Check sheet for the modelled part. Datum: model origin and axes. Units: mm. Face numbers are marked on the shaded views. A direction names the side the tool comes from. Give positions to 0.01 mm unless a question says otherwise; leave off trailing zeros. Order: outer loops, then holes, each group sorted by start corner. A loop starts at its lowest first (then second) coordinate and runs counter-clockwise, first axis right, second up.
Autodesk Inventor part; units mm, degrees
ref_plane "YZ Plane" through (0, 0, 0) normal (1, 0, 0) x (0, 1, 0)
ref_plane "XZ Plane" through (0, 0, 0) normal (0, 1, 0) x (-1, 0, 0)
ref_plane "XY Plane" through (0, 0, 0) normal (0, 0, 1) x (1, 0, 0)
sketch "Sketch1" plane through (0, 0, 0) normal (0, 1, 0) x (-1, 0, 0)
  line L0 (-40, -47.5) -> (40, -47.5)
  line L1 (40, -47.5) -> (40, 47.5)
  line L2 (40, 47.5) -> (-40, 47.5)
  line L3 (-40, 47.5) -> (-40, -47.5)
  line L4 (-40, -47.5) -> (40, 47.5) construction
  line L5 (40, -47.5) -> (-40, 47.5) construction
  line L6 (25.5, 17) -> (28.5, 17)
  line L7 (0, 17.5) -> (0, 19)
  line L8 (0, 0) -> (2.25, 0)
  line L9 (0, 0) -> (0, 17.5)
  line L10 (-27.5, -36.75) -> (-27.5, 38.25)
  line L11 (-27.5, 38.25) -> (28.5, -36.75) construction
  line L12 (28.5, 38.25) -> (-27.5, -36.75) construction
  line L13 (28.5, 38.25) -> (28.5, -36.75)
  line L14 (28.5, 17) -> (28.5, -36.75)
  line L15 (28.5, -36.75) -> (-27.5, -36.75)
  line L16 (0, -31.5) -> (8.5, -31.5)
  line L17 (0, 0) -> (0, -31.5)
  line L18 (0, -31.5) -> (-19.5, -31.5)
  line L19 (-19.5, -31.5) -> (-19.5, -36.75)
  line L20 (-27.5, 38.25) -> (28.5, 38.25)
  line L21 (0, 19) -> (24, 19)
  line L22 (0, 0) -> (0, 31.5)
  line L23 (28.5, -17) -> (28.5, 36.75)
  line L24 (28.5, -38.25) -> (28.5, 36.75)
  line L25 (28.5, -38.25) -> (-27.5, 36.75) construction
  line L26 (-27.5, 36.75) -> (-27.5, -38.25)
  line L27 (-27.5, -38.25) -> (28.5, 36.75) construction
  line L28 (0, 31.5) -> (8.5, 31.5)
  circle A0 centre (8.5, 31.5) radius 2.5
  line L29 (0, 31.5) -> (-19.5, 31.5)
  circle A1 centre (-19.5, 31.5) radius 2.5
  circle A2 centre (-19.5, 31.5) radius 2.5
  line L30 (-19.5, 31.5) -> (-19.5, 36.75)
  line L31 (28.5, 36.75) -> (-27.5, 36.75)
  line L32 (0, 0) -> (0, -17.5)
  line L33 (0, -17.5) -> (0, -19)
  line L34 (25.5, -17) -> (28.5, -17)
  line L35 (0, -19) -> (24, -19)
  line L36 (-27.5, -38.25) -> (28.5, -38.25)
  circle A3 centre (24, -19) radius 2.5
  point P0 (0.5, 0.75)
  point P1 (0.5, -0.75)
  dimension "d0" = 80
  dimension "d1" = 95
  dimension "d5" = 17.5
  dimension "d6" = 8.5
  dimension "d7" = 19.5
  dimension "d8" = 31.5
  dimension "d9" = 24
  dimension "d11" = 2.25
  dimension "d12" = 56
  dimension "d13" = 75
  dimension "d14" = 5.25
  dimension "d15" = 3
ref_plane "Work Plane3" through (0, 10, 0) normal (0, 1, 0) x (1, 0, 0)
sketch "Sketch2" plane through (0, 10, 0) normal (0, 1, 0) x (1, 0, 0)
  line L0 (35.5, -47.5) -> (40, -39.7058)
  line L1 (35.5, -47.5) -> (44.5, -47.5) construction
  line L2 (40, -39.7058) -> (35.5, -39.7058)
  line L3 (35.5, -39.7058) -> (35.5, -47.5)
  line L4 (-40, -47.5) -> (40, -47.5)
  line L5 (40, -47.5) -> (40, 47.5)
  line L6 (40, -37.7058) -> (33.5, -37.7058)
  line L7 (33.5, -37.7058) -> (33.5, -47.5)
  line L8 (33.5, -47.5) -> (35.5, -47.5)
  line L9 (40, -39.7058) -> (40, -37.7058)
  line L10 (0, -47.5) -> (0, 47.5)
  line L11 (-35.5, -47.5) -> (-40, -39.7058)
  line L12 (-35.5, -47.5) -> (-44.5, -47.5) construction
  line L13 (-40, -39.7058) -> (-35.5, -39.7058)
  line L14 (-35.5, -39.7058) -> (-35.5, -47.5)
  line L15 (-40, -37.7058) -> (-33.5, -37.7058)
  line L16 (-33.5, -37.7058) -> (-33.5, -47.5)
  line L17 (-33.5, -47.5) -> (-35.5, -47.5)
  line L18 (-40, -39.7058) -> (-40, -37.7058)
  line L19 (40, 47.5) -> (-40, 47.5)
  line L20 (-40, 47.5) -> (-33.5, 47.5)
  line L21 (-33.5, 47.5) -> (-33.5, 37.5)
  line L22 (-33.5, 37.5) -> (-40, 37.5)
  line L23 (-40, 37.5) -> (-40, 47.5)
  line L24 (40, 47.5) -> (33.5, 47.5)
  line L25 (33.5, 47.5) -> (33.5, 37.5)
  line L26 (33.5, 37.5) -> (40, 37.5)
  line L27 (40, 37.5) -> (40, 47.5)
  point P0 (0, 0)
  dimension "d18" = 9
  dimension "d19" = 60
  dimension "d20" = 2
  dimension "d21" = 9.7942
  dimension "d22" = 6.5
  dimension "d23" = 6.5
  dimension "d24" = 10
  dimension "d25" = 6.5
  dimension "d26" = 10
extrude "Extrusion2" add sketch "Sketch2" along normal blind 100 contours L3 L2 L0 | L4 L7 L6 L5 L2 L3 | L26 L25 L19 L5 | L14 L13 L18 L15 L16 L4 | L11 L13 L14 | L21 L22 L23 L19
ref_plane "Work Plane2" through (0, 10, 0) normal (0, 1, 0) x (1, 0, 0)
sketch "Sketch3" plane through (0, 10, 0) normal (0, 1, 0) x (1, 0, 0)
  line L0 (-40, 37.5) -> (-40, -37.7058)
  line L1 (-33.5, 37.5) -> (-40, 37.5)
  line L2 (-40, -37.7058) -> (-36.75, -37.7058)
  line L3 (-36.75, -37.7058) -> (-36.75, 37.5)
  line L4 (-36.75, 37.5) -> (-40, 37.5)
  line L5 (-40, 37.5) -> (-40, -37.7058)
  line L6 (33.5, 37.5) -> (40, 37.5)
  line L7 (40, -37.7058) -> (33.5, -37.7058)
  line L8 (40, 37.5) -> (36.75, 37.5)
  line L9 (36.75, 37.5) -> (36.75, -37.7058)
  line L10 (36.75, -37.7058) -> (40, -37.7058)
  line L11 (40, -37.7058) -> (40, 37.5)
  point P0 (0, 0)
extrude "Extrusion3" add sketch "Sketch3" along normal blind 5
ref_plane "Work Plane4" through (0, 110, 0) normal (0, 1, 0) x (1, 0, 0)
sketch "Sketch4" plane through (0, 110, 0) normal (0, 1, 0) x (1, 0, 0)
  line L0 (-33.5, 47.5) -> (-40, 47.5)
  line L1 (-40, -47.5) -> (40, -47.5)
  line L2 (-40, 47.5) -> (-33.5, 47.5)
  line L3 (-33.5, 47.5) -> (-33.5, -47.5)
  line L4 (-33.5, -47.5) -> (-40, -47.5)
  line L5 (-40, -47.5) -> (-40, 47.5)
  line L6 (40, 37.5) -> (40, 47.5)
  line L7 (40, 47.5) -> (33.5, 47.5)
  line L8 (33.5, 47.5) -> (33.5, -47.5)
  line L9 (33.5, -47.5) -> (40, -47.5)
  line L10 (40, -47.5) -> (40, 47.5)
  line L11 (40, -37.7058) -> (33.5, -37.7058)
  line L12 (33.5, -37.7058) -> (-33.5, -37.7058)
  line L13 (-33.5, -37.7058) -> (-33.5, -47.5)
  line L14 (-33.5, -47.5) -> (33.5, -47.5)
  line L15 (33.5, -47.5) -> (33.5, -37.7058)
  point P0 (0, 0)
extrude "Extrusion4" add sketch "Sketch4" along normal blind 8
ref_plane "Work Plane8" through (40, 0, -47.5) normal (0, 0, -1) x (-1, 0, 0)
sketch "Sketch5" plane through (40, 0, -47.5) normal (0, 0, -1) x (-1, 0, 0)
  line L0 (73.5, 110) -> (6.5, 110)
  line L1 (6.5, 110) -> (6.5, 113)
  line L2 (6.5, 10) -> (6.5, 118)
  line L3 (6.5, 113) -> (3.25, 113)
  line L4 (3.25, 113) -> (3.25, 116)
  line L5 (3.25, 116) -> (6.5, 116)
  line L6 (6.5, 116) -> (6.5, 113)
  line L7 (73.5, 10) -> (73.5, 118)
  line L8 (6.5, 116) -> (73.5, 116)
  line L9 (73.5, 116) -> (73.5, 113)
  line L10 (73.5, 113) -> (6.5, 113)
  line L11 (6.5, 113) -> (6.5, 116)
  line L12 (73.5, 113) -> (76.75, 113)
  line L13 (76.75, 113) -> (76.75, 116)
  line L14 (76.75, 116) -> (73.5, 116)
  line L15 (73.5, 116) -> (73.5, 113)
  point P0 (40, 0)
  dimension "d33" = 3
  dimension "d34" = 3
  dimension "d35" = 3.25
  dimension "d36" = 3.25
extrude "Extrusion5" cut sketch "Sketch5" against normal blind 90.206 contours L10 L2 L8 L7 | L7 L14 L13 L12 | L3 L4 L5 L2
ref_plane "Work Plane7" through (40, 10, 39.7058) normal (0.8660254, 0, 0.5) x (0.5, 0, -0.8660254)
sketch "Sketch6" plane through (40, 10, 39.7058) normal (0.8660254, 0, 0.5) x (0.5, 0, -0.8660254)
  line L0 (-9, 0) -> (-9, 100)
  line L1 (0, 0) -> (-9, 0)
  line L2 (-9, 100) -> (0, 100)
  line L3 (0, 100) -> (0, 0)
  line L4 (0, 0) -> (-9, 0)
  line L5 (-9, 0) -> (-9, 100)
  line L6 (0, 100) -> (0, 70)
  line L7 (0, 0) -> (0, 100)
  line L8 (0, 70) -> (-4.5, 70)
  circle A0 centre (-4.5, 70) radius 1.5
  point P0 (14.3862, -10)
  dimension "d39" = 30
  dimension "d40" = 3
extrude "Extrusion6" cut sketch "Sketch6" against normal blind 6 contours A0
ref_plane "Work Plane6" through (-35.5, 10, 47.5) normal (-0.8660254, 0, 0.5) x (0.5, 0, 0.8660254)
sketch "Sketch7" plane through (-35.5, 10, 47.5) normal (-0.8660254, 0, 0.5) x (0.5, 0, 0.8660254)
  line L0 (-9, 0) -> (-9, 100)
  line L1 (0, 0) -> (0, 100)
  line L2 (-9, 100) -> (0, 100)
  line L3 (0, 100) -> (0, 0)
  line L4 (0, 0) -> (-9, 0)
  line L5 (-9, 0) -> (-9, 100)
  line L6 (-9, 100) -> (-9, 70)
  line L7 (-9, 70) -> (-4.5, 70)
  circle A0 centre (-4.5, 70) radius 1.5
  point P0 (-23.3862, -10)
  dimension "d43" = 30
  dimension "d44" = 3
extrude "Extrusion7" cut sketch "Sketch7" against normal blind 6 contours A0
ref_plane "Work Plane5" through (40, 0, 47.5) normal (1, 0, 0) x (0, 0, -1)
sketch "Sketch8" plane through (40, 0, 47.5) normal (1, 0, 0) x (0, 0, -1)
  line L0 (85, 110) -> (9.7942, 110)
  line L1 (85, 110) -> (95, 110)
  line L2 (95, 110) -> (95, 80)
  line L3 (95, 80) -> (85, 80)
  line L4 (85, 80) -> (85, 110)
  circle A0 centre (90, 80) radius 1.5
  point P0 (47.5, 0)
  dimension "d47" = 10
  dimension "d48" = 30
  dimension "d49" = 3
extrude "Extrusion8" [suppressed]
ref_plane "Work Plane1" through (0, 0, 0) normal (0, -1, 0) x (1, 0, 0)
sketch "Sketch9" plane through (0, 0, 0) normal (0, -1, 0) x (1, 0, 0)
  line L0 (40, 47.5) -> (40, 39.7058)
  line L1 (40, 47.5) -> (25, 47.5)
  line L2 (25, 47.5) -> (25, -10)
  line L3 (25, -10) -> (40, -10)
  line L4 (40, -10) -> (40, 47.5)
  line L5 (-40, 47.5) -> (-35.5, 47.5)
  line L6 (-40, 47.5) -> (-25, 47.5)
  line L7 (-25, 47.5) -> (-25, -10)
  line L8 (-25, -10) -> (-40, -10)
  line L9 (-40, -10) -> (-40, 47.5)
  line L10 (-40, 47.5) -> (40, 47.5)
  line L11 (-40, 47.5) -> (-32.5, 47.5)
  line L12 (-33.5, 47.5) -> (-33.5, 37.7058)
  line L13 (-40, 47.5) -> (-33.5, 47.5)
  line L14 (-33.5, 47.5) -> (-29, 47.5)
  line L15 (-40, 47.5) -> (-32.5, 47.5)
  line L16 (-32.5, 47.5) -> (-32.5, 32.5)
  circle A0 centre (-32.5, 32.5) radius 3
  line L17 (-32.5, -10) -> (-32.5, -25)
  circle A1 centre (-32.5, -25) radius 3
  line L18 (32.5, 47.5) -> (32.5, 32.5)
  line L19 (32.5, -10) -> (32.5, -25)
  circle A2 centre (32.5, -25) radius 3
  circle A3 centre (32.5, 32.5) radius 3
  point P0 (0, 0)
  dimension "d52" = 15
  dimension "d53" = 57.5
  dimension "d54" = 15
  dimension "d55" = 57.5
  dimension "d61" = 7.5
  dimension "d62" = 15
  dimension "d63" = 6
  dimension "d64" = 15
  dimension "d65" = 6
  dimension "d66" = 15
  dimension "d67" = 15
  dimension "d68" = 6
  dimension "d69" = 6
extrude "Extrusion9" add sketch "Sketch1" along normal blind 10 contours L3 L2 L1 L0 | L9 L17 L18 L19 L15 L10 L31 L30 A1 L29 L22 L7 | L7 L22 L29 A1 L30 L31 L13 L34 A3 L35 L17 L9 | L35 A3 L34 L13 L15 L19 L18 L17 | L31 L10 L20 L13 | L15 L24 L36 L26
extrude "Extrusion11" cut sketch "Sketch9" against normal up to surface (10 mm away) contours A0 | A1 | A2 | A3
equation "\"d72\" = d68"
properties part number "Base"
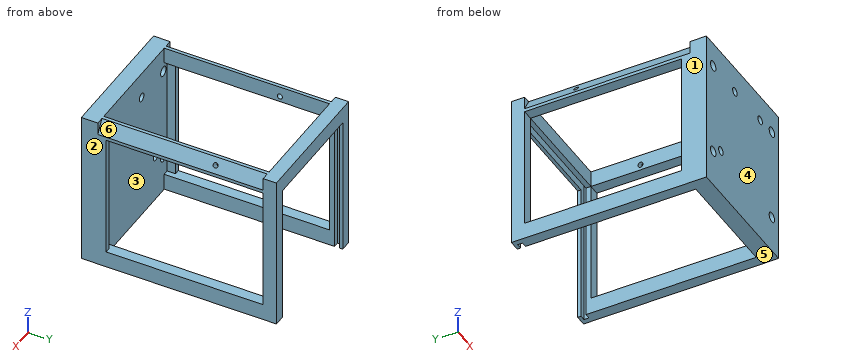
(1) Cross-section at B-B on y = 104. Enter the section's corners in (x, z), then the cut area to 3 significant figures.
Response values:
outline: (-40, -47.5) - (-33.5, -47.5) - (-33.5, -37.5) - (-40, -37.5) - close; (-40, 37.71) - (-33.5, 37.71) - (-33.5, 47.5) - (-35.5, 47.5) - (-40, 39.71) - close; (33.5, -47.5) - (40, -47.5) - (40, -37.5) - (33.5, -37.5) - close; (33.5, 37.71) - (40, 37.71) - (40, 39.71) - (35.5, 47.5) - (33.5, 47.5) - close
area: 222 mm2
(2) Cross-section at D-D on z = 24. Enter the section's corners in (x, y).
Response values:
outline: (-40, 0) - (40, 0) - (40, 15) - (36.75, 15) - (36.75, 10) - (-36.75, 10) - (-36.75, 15) - (-40, 15) - close; (-40, 110) - (-33.5, 110) - (-33.5, 113) - (-36.75, 113) - (-36.75, 116) - (-33.5, 116) - (-33.5, 118) - (-40, 118) - close; (33.5, 110) - (40, 110) - (40, 118) - (33.5, 118) - (33.5, 116) - (36.75, 116) - (36.75, 113) - (33.5, 113) - close
(3) Cross-section at C-C on z = -19. Enter the section's corners in (x, y), then the cut area to 3 significant figures.
Response values:
outline: (-40, 0) - (-26.5, 0) - (-26.5, 10) - (-36.75, 10) - (-36.75, 15) - (-40, 15) - close; (-40, 110) - (-33.5, 110) - (-33.5, 113) - (-36.75, 113) - (-36.75, 116) - (-33.5, 116) - (-33.5, 118) - (-40, 118) - close; (-21.5, 0) - (40, 0) - (40, 15) - (36.75, 15) - (36.75, 10) - (-21.5, 10) - close; (33.5, 110) - (40, 110) - (40, 118) - (33.5, 118) - (33.5, 116) - (36.75, 116) - (36.75, 113) - (33.5, 113) - close
area: 867 mm2
(4) Gauge pin test, flat ends, axial feed: pin 1 Ø12 at (x, z) = (31, 33.5) entering from -Y; pin 2 Ø6 at (x, z) = (-6.5, -9) entering from +Y; pin 3 Ø12 at (y, z) = (91, 30.5) entering from -X; pin 4 Ø0.9 at (x, y) = (-4.5, 111.5) entering from -Z. Record the tip position at first contact, or that the pin passes through.
Response values:
pin 1: stops at y = 0
pin 2: stops at y = 10
pin 3: passes through
pin 4: stops at z = 37.71
(5) Release check for a two-part mould opening along X. For the marked faces 1, 2, 3 and 4 record: released by +X, released by -X, zero draft, split by the parting line, or undercut.
Response values:
face 1: released by -X
face 2: released by +X
face 3: undercut
face 4: zero draft
(6) Set-up check for the marked faces 5 and 6: record each of +Z, -Z, +X, -X, +Y, -Y from which the full face is reachable in a straight line by a thin tool's end or side.
Response values:
face 5: -Z, +X, -X, +Y, -Y
face 6: +Z, +X
(7) Cross-section at A-A on x = 10. Enter the section's corners in (y, z).
Response values:
outline: (0, -47.5) - (10, -47.5) - (10, 47.5) - (0, 47.5) - close; (110, 37.71) - (113, 37.71) - (113, 42.71) - (116, 42.71) - (116, 37.71) - (118, 37.71) - (118, 47.5) - (110, 47.5) - close
(8) Material ranges on L1, parallel to Y at x = -35.5, z = 2.5; L2, parallel to Z at x = -32.5, y = 7.5; L3, parallel to X at y = 7.25, z = 32.5, recorded low to high.
Response values:
L1: y = 0 to 10, 110 to 113, 116 to 118
L2: z = -47.5 to -28, -22 to 29.5, 35.5 to 47.5
L3: x = -40 to -35.5, -29.5 to -10.79, -6.21 to 17.21, 21.79 to 29.5, 35.5 to 40
